Model file for the job. Use its own axes, mm. A direction names the side the tool comes from. Give positions to 0.01 mm unless a question says otherwise; leave off trailing zeros. Loops run counter-clockwise (first coordinate to the right, second up) from the corner with the lowest first, then second, coordinate; pieces in that order, holes last. Notation, with made-up numbers: (75, 28) - (98, 28) arc R27 ccw to (98, 46) - close; hole circle Ø7 at (-7, 41). An arc over 180 degrees is marked (long way). Use a Markdown table: item, result.
from build123d import *

# Parameters (mm, degrees)
F0_R     = 11
F0_R_2   = 4
F1_DEPTH = 10
F2_R     = 10
F2_R_2   = 4
F3_DEPTH = 5
F4_R     = 11
F4_R_2   = 10
F4_R_3   = 4
F5_DEPTH = 5


# Not quite as in the source:
# - a fillet or chamfer that OpenCascade refuses, or shapes differently, is made with other operations: its cross-section is extruded or revolved along the edge and cut away or added


with BuildPart() as f1:
    # F0 (on Top) → F1 (new body)
    with BuildSketch(Plane.XY):
        Circle(F0_R)
        with Locations((-0.2262097114, 0)):
            Circle(F0_R_2, mode=Mode.SUBTRACT)
    extrude(amount=F1_DEPTH)

    # F2 (on face) → F3 (join)
    with BuildSketch(Plane.XY.offset(10)):
        Circle(F2_R)
        with Locations((-0.2262097114, 0)):
            Circle(F2_R_2, mode=Mode.SUBTRACT)
    extrude(amount=F3_DEPTH)

    # F4 (on face) → F5 (join)
    with BuildSketch(Plane.XY.offset(15)):
        Circle(F4_R)
        Circle(F4_R_2, mode=Mode.SUBTRACT)
        Circle(F4_R_2)
        with Locations((-0.2262097114, 0)):
            Circle(F4_R_3, mode=Mode.SUBTRACT)
    extrude(amount=F5_DEPTH)

    # F6: fillet of radius 3 on 2 edges, made by hand

    # F6_s1 → F6_t2 (revolve, cut)
    with BuildSketch(Plane.XZ):
        with BuildLine():
            ThreePointArc((10, 15), (10.7386127875, 16.0113231061), (11, 17.2360679775))
            Line((11, 17.2360679775), (11, 15))
            Line((11, 15), (10, 15))
        make_face()
    revolve(axis=Axis((0, 0, 15), (0, 0, 1)), mode=Mode.SUBTRACT)

    # F6_s3 → F6_t4 (revolve, cut)
    with BuildSketch(Plane.XZ):
        with BuildLine():
            ThreePointArc((11, 7.7639320225), (10.7386127875, 8.9886768939), (10, 10))
            Line((10, 10), (11, 10))
            Line((11, 10), (11, 7.7639320225))
        make_face()
    revolve(axis=Axis((0, 0, 10), (0, 0, 1)), mode=Mode.SUBTRACT)

    # F7: fillet of radius 5 on 1 edges, made by hand

    # F7_s1 → F7_t2 (revolve, cut)
    with BuildSketch(Plane.XZ):
        with BuildLine():
            ThreePointArc((6.527864045, 20), (9.1565196056, 19.2532540418), (11, 17.2360679775))
            Line((11, 17.2360679775), (11, 20))
            Line((11, 20), (6.527864045, 20))
        make_face()
    revolve(axis=Axis((0, 0, 20), (0, 0, 1)), mode=Mode.SUBTRACT)


solid = f1.part
(1) Slice it at C-C, the plane z = 2.5. Write the cut outline in (x, y).
Computed:
| item | result |
|---|---|
| outline | circle Ø22 at (0, 0); hole circle Ø8 at (-0.23, 0) |
(2) 3-axis set-ups, long thin cutter, end or side, ignore diameter. For faces 4 (the cylindrical face through (-2.17, -9.76, 12.46)), 5 (the flat face through (3, -3, 20)): which of +Z, -Z, +X, -X, +Y, -Y reach the whole face in a straight line?
Computed:
| item | result |
|---|---|
| face 4 | none |
| face 5 | +Z, +X, -X, +Y, -Y |
(3) Drill centre lines: probe 1 along X at (y, z) = (2.75, 13.5); probe 2 along Z at (x, y) = (-5.5, 9.25); probe 3 along Y at (x, z) = (-1.75, 15.75). Where is each one in solid material? Low to high. Write a range as [from, to].
Computed:
| item | result |
|---|---|
| probe 1 | [-9.61, -3.13], [2.68, 9.61] |
| probe 2 | [0, 8.94], [16.06, 17.66] |
| probe 3 | [-10.46, -3.7], [3.7, 10.46] |
(4) Mould opens along Y. For faces 1 (the cylindrical face through (-2.38, -10.74, 3.83)), 2 (the cylindrical face through (-1.093, -3.905, 9.86)), 3 (the flat face through (0, -5, 0)) say: pulls with the +Y half, pulls with the -Y half, needs draft (parallel to the pull), parting line crosses it, or undercut.
Computed:
| item | result |
|---|---|
| face 1 | parting line crosses it |
| face 2 | undercut |
| face 3 | needs draft |
(5) Slice it at A-A, the plane y = 0. Write the cut outline in (x, z).
Computed:
| item | result |
|---|---|
| outline | (-11, 0) - (-4.23, 0) - (-4.23, 20) - (-6.53, 20) arc R5 ccw to (-11, 17.24) arc R3 ccw to (-10, 15) - (-10, 10) arc R3 ccw to (-11, 7.76) - close; (3.77, 0) - (11, 0) - (11, 7.76) arc R3 ccw to (10, 10) - (10, 15) arc R3 ccw to (11, 17.24) arc R5 ccw to (6.53, 20) - (3.77, 20) - close |
(6) Slice it at B-B, the plane x = 0. Write the cut outline in (y, z).
Computed:
| item | result |
|---|---|
| outline | (-11, 0) - (-3.99, 0) - (-3.99, 20) - (-6.53, 20) arc R5 ccw to (-11, 17.24) arc R3 ccw to (-10, 15) - (-10, 10) arc R3 ccw to (-11, 7.76) - close; (3.99, 0) - (11, 0) - (11, 7.76) arc R3 ccw to (10, 10) - (10, 15) arc R3 ccw to (11, 17.24) arc R5 ccw to (6.53, 20) - (3.99, 20) - close |
(7) Pin check, flat tips, straight feed: P1, Ø1.5, axis at x = 0.5, z = 15, coming from the +Y side; P2, Ø1.5, axis at x = -8, z = 12, coming from the -Y side; P3, Ø3, axis at y = 7.5, z = 5.5, coming from the -X side. Stop position of each tip, or through.
Computed:
| item | result |
|---|---|
| P1 | y = 10.6 |
| P2 | y = -6.89 |
| P3 | x = -9.22 |
